Model file for the job. Use its own axes, mm. Face numbers are marked on the shaded views. A direction names the side the tool comes from. Coordinates: 2 decimals unless noted, no trailing zeros. Write each loop counter-clockwise with the first axis right and the second up, starting at its lowest first coordinate (ties: lowest second). Pieces come first, ordered by that corner, then holes.
Q1. Band-saw the part on B-B, the plane z = 2.75. Write the cut outline in (x, y), plus the area to 3 significant figures.
Q2. Pin check, flat tips, straight feed: P1, Ø0.9, axis at y = 5.5, z = 4.5, coming from the +X side; P2, Ø0.9, axis at y = 5.5, z = 3, coming from the -X side. Stop position of each tip, or through.
Q3. Which spindle directions (+Z, -Z, +X, -X, +Y, -Y) get a long thin tool onto all of the face, cutting with end or side? Do the marked faces 4 and 5. Say none if no direction does.
Q4. Drill centre lines: probe 1 along Y at (x, z) = (0, 2.75); probe 2 along X at (y, z) = (6, 0.5); probe 3 along X at (y, z) = (-1.75, 5). Where is each one in solid material? Low to high.
Q5. Pull direction Y, two halves, no side cores. Call the marked faces 1, 2 and 3: released by +Y, released by -Y, zero draft, split by the parting line, or undercut.
Q6. Band-saw the part on C-C, the plane y = 0.75. Write the cut outline in (x, z), plus the area to 3 significant figures.
Q7. Band-saw the part on D-D, the plane y = -4. Write the cut outline in (x, z).
Q8. Band-saw the part on A-A, the plane x = 0. Write the cut outline in (y, z).
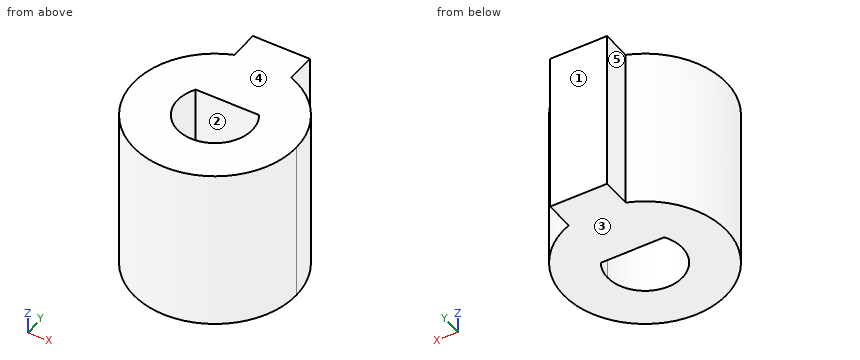
from build123d import *

# Parameters (mm, degrees)
BOSS_EXTRUDE1_DEPTH = 10


with BuildPart() as part:
    # Sketch2 → Boss-Extrude1 (new body)
    with BuildSketch(Plane.XY):
        with BuildLine():
            ThreePointArc((0, 5), (0.889173073, 4.920301947), (1.75, 4.683748499))
            Line((1.75, 4.683748499), (1.75, 6.5))
            Line((1.75, 6.5), (0, 6.5))
            Line((0, 6.5), (0, 5))
        make_face()
        with BuildLine():
            ThreePointArc((-1.75, 4.683748499), (-0.889173073, 4.920301947), (0, 5))
            Line((0, 5), (0, 6.5))
            Line((0, 6.5), (-1.75, 6.5))
            Line((-1.75, 6.5), (-1.75, 4.683748499))
        make_face()
        with BuildLine():
            ThreePointArc((1.75, 1.492481156), (1.856113866, 1.358249358), (1.95195478, 1.216500118))
            ThreePointArc((1.95195478, 1.216500118), (2.211277458, 0.632654726), (2.3, 0))
            ThreePointArc((2.3, 0), (-0.632654726, -2.211277458), (-1.95195478, 1.216500118))
            ThreePointArc((-1.95195478, 1.216500118), (-1.856113866, 1.358249358), (-1.75, 1.492481156))
            Line((-1.75, 1.492481156), (-1.75, 4.683748499))
            ThreePointArc((-1.75, 4.683748499), (-2.850438563, -4.107919181), (5, 0))
            ThreePointArc((5, 0), (4.107919181, 2.850438563), (1.75, 4.683748499))
            Line((1.75, 4.683748499), (1.75, 1.492481156))
        make_face()
        with BuildLine():
            ThreePointArc((-1.75, 1.492481156), (-0.963663152, 2.08838534), (0, 2.3))
            Line((0, 2.3), (0, 5))
            ThreePointArc((0, 5), (-0.889173073, 4.920301947), (-1.75, 4.683748499))
            Line((-1.75, 4.683748499), (-1.75, 1.492481156))
        make_face()
        with BuildLine():
            ThreePointArc((0, 2.3), (0.963663152, 2.08838534), (1.75, 1.492481156))
            Line((1.75, 1.492481156), (1.75, 4.683748499))
            ThreePointArc((1.75, 4.683748499), (0.889173073, 4.920301947), (0, 5))
            Line((0, 5), (0, 2.3))
        make_face()
        with BuildLine():
            Line((0, 1.216500118), (1.75, 1.216500118))
            Line((1.75, 1.216500118), (1.75, 1.492481156))
            ThreePointArc((1.75, 1.492481156), (0.963663152, 2.08838534), (0, 2.3))
            Line((0, 2.3), (0, 1.216500118))
        make_face()
        with BuildLine():
            Line((-1.75, 1.216500118), (0, 1.216500118))
            Line((0, 1.216500118), (0, 2.3))
            ThreePointArc((0, 2.3), (-0.963663152, 2.08838534), (-1.75, 1.492481156))
            Line((-1.75, 1.492481156), (-1.75, 1.216500118))
        make_face()
        with BuildLine():
            ThreePointArc((-1.75, 1.492481156), (-1.856113866, 1.358249358), (-1.95195478, 1.216500118))
            Line((-1.95195478, 1.216500118), (-1.75, 1.216500118))
            Line((-1.75, 1.216500118), (-1.75, 1.492481156))
        make_face()
        with BuildLine():
            Line((1.75, 1.216500118), (1.95195478, 1.216500118))
            ThreePointArc((1.95195478, 1.216500118), (1.856113866, 1.358249358), (1.75, 1.492481156))
            Line((1.75, 1.492481156), (1.75, 1.216500118))
        make_face()
    extrude(amount=BOSS_EXTRUDE1_DEPTH)


solid = part.part
Answer sheet:
1. outline: (-1.75, 4.68) arc R5 ccw (long way) to (1.75, 4.68) - (1.75, 6.5) - (-1.75, 6.5) - close; hole (-1.95, 1.22) arc R2.3 ccw (long way) to (1.95, 1.22) - close
1. area: 70.5 mm2
2. P1: stops at x = 1.75
2. P2: stops at x = -1.75
3. face 4: +Z, +X, -X, +Y, -Y
3. face 5: +Z, -Z, -X, +Y
4. probe 1: y = -5 to -2.3, 1.22 to 6.5
4. probe 2: x = -1.75 to 1.75
4. probe 3: x = -4.68 to -1.49, 1.49 to 4.68
5. face 1: released by +Y
5. face 2: undercut
5. face 3: zero draft
6. outline: (-4.94, 0) - (-2.17, 0) - (-2.17, 10) - (-4.94, 10) - close; (2.17, 0) - (4.94, 0) - (4.94, 10) - (2.17, 10) - close
6. area: 55.4 mm2
7. outline: (-3, 0) - (3, 0) - (3, 10) - (-3, 10) - close
8. outline: (-5, 0) - (-2.3, 0) - (-2.3, 10) - (-5, 10) - close; (1.22, 0) - (6.5, 0) - (6.5, 10) - (1.22, 10) - close
